Input: part model. Units: mm. Frame: model coordinates. A direction names the side the tool comes from. Round coordinates to 2 decimals unless told otherwise and drop trailing zeros. Loops run counter-clockwise (first coordinate to the right, second up) from the corner with the lowest first, then second, coordinate; pieces in that order, holes last. Notation, with made-up numbers: (45.5, 40.25) - (76.5, 40.25) arc R28 cw to (76.5, 79.25) - close; hole circle Ø8 at (-31, -33.75). An arc over 180 degrees is marked (long way). Use CSV: the item, a comma, the result in double quotes. Start each with the question number.
1. Material intervals for probe 1 along X at (y, z) = (40.5, 3.4); probe 2 along Y at (x, z) = (111.5, 3.4); probe 3 along Y at (x, z) = (22.5, 1.1), sorted ascending. Write a range as from..to.
2. Cut plane A-A (y = 37). Return loops of the section in (x, z), and give its area (3 significant figures).
3. Access query for faces 5 (the flat face through (135, -4.8, 3)), 6 (the flat face through (120, 42, 3)), 7 (the flat face through (128.725, 19.699, 2.465)). Directions: +Z, -Z, +X, -X, +Y, -Y. A direction counts if a zero-diameter tool reaches every point of the face in a straight line with its end or side. Return the directions, or none.
4. Cut plane C-C (x = 137.5). Return loops of the section in (y, z), and give its area (3 significant figures).
5. Cut plane B-B (x = 83.5). Return loops of the section in (y, z), and give its area (3 significant figures).
6. Pull-direction query (Y, two-part tool) for faces 1 (the flat face through (45, 0, 2)), 2 (the cylindrical face through (13.3, 35.5, 2.5)), 3 (the flat face through (30, 42, 3)), 4 (the flat face through (105, 40, 2)); classes: +Y half, -Y half, draft (parallel to the pull), parting line (faces both ways), or undercut.
7. Pin query (flat end, axial travel): P1, Ø2, axis at x = 32.5, z = 4.5, coming from the -Y side; P2, Ø1.5, axis at x = 105, z = 3.5, coming from the +Y side. Return the tip coordinate at first contact, or that it passes through.
8. Cut plane D-D (z = 3.75). Give the number of separate pieces and of enclosed holes in the cut face, and give its area (3 significant figures).
```python
from build123d import *

# Parameters (mm, degrees)
SKETCH_1_W          = 150
SKETCH_1_H          = 40
EXTRUDE_1_DEPTH     = 5
SKETCH_2_W          = 30
SKETCH_2_H          = 4.8
EXTRUDE_2_DEPTH     = 5
SKETCH_3_R          = 1.1
CUT_EXTRUDE_1_DEPTH = 5
FILLET_1_R          = 1
CUT_EXTRUDE_2_DEPTH = 10
FILLET_2_R          = 1.1
HOLE_WIZARD_M3_1_D  = 3.4


with BuildPart() as part:
    # 草图1 → 凸台-拉伸1 (new body)
    with BuildSketch(Plane.XY):
        with Locations((75, 20)):
            Rectangle(SKETCH_1_W, SKETCH_1_H)
    extrude(amount=EXTRUDE_1_DEPTH)

    # 草图2 → 凸台-拉伸2 (add)
    with BuildSketch(Plane.XY.offset(5)):
        with Locations((15, 42.4)):
            Rectangle(SKETCH_2_W, SKETCH_2_H)
        with Locations((75, 42.4)):
            Rectangle(SKETCH_2_W, SKETCH_2_H)
        with Locations((135, 42.4)):
            Rectangle(SKETCH_2_W, SKETCH_2_H)
        with Locations((15, -2.4)):
            Rectangle(SKETCH_2_W, SKETCH_2_H)
        with Locations((75, -2.4)):
            Rectangle(SKETCH_2_W, SKETCH_2_H)
        with Locations((135, -2.4)):
            Rectangle(SKETCH_2_W, SKETCH_2_H)
    extrude(amount=-EXTRUDE_2_DEPTH)

    # 草图3 → 切除-拉伸1 (cut)
    with BuildSketch(Plane.XY.offset(5)):
        with Locations((30, 40)):
            Circle(SKETCH_3_R)
        with Locations((60, 40)):
            Circle(SKETCH_3_R)
        with Locations((90, 40)):
            Circle(SKETCH_3_R)
        with Locations((120, 40)):
            Circle(SKETCH_3_R)
        with Locations((30, 0)):
            Circle(SKETCH_3_R)
        with Locations((60, 0)):
            Circle(SKETCH_3_R)
        with Locations((90, 0)):
            Circle(SKETCH_3_R)
        with Locations((120, 0)):
            Circle(SKETCH_3_R)
    extrude(amount=-CUT_EXTRUDE_1_DEPTH, mode=Mode.SUBTRACT)

    # 圆角1
    fillet_1_edges = [part.edges().sort_by_distance(p)[0] for p in [
        (0, 44.8, 2.5),
        (30, 44.8, 2.5),
        (60, 44.8, 2.5),
        (90, 44.8, 2.5),
        (150, 44.8, 2.5),
        (120, 44.8, 2.5),
        (0, -4.8, 2.5),
        (30, -4.8, 2.5),
        (60, -4.8, 2.5),
        (90, -4.8, 2.5),
        (120, -4.8, 2.5),
        (150, -4.8, 2.5),
    ]]
    fillet(fillet_1_edges, radius=FILLET_1_R)

    # 草图5 → 切除-拉伸2 (cut)
    with BuildSketch(Plane(origin=(0, 0, 0), x_dir=(-1, 0, 0), z_dir=(0, 0, -1))):
        Polygon((-114.766536075, 32), (-118.9, 32), (-142, 32), (-142, 8), align=None)
        Polygon((-102.666666667, 8), (-102.666666667, 32), (-129.900130591, 8), align=None)
        Polygon((-67.433202742, 8), (-94.666666667, 32), (-94.666666667, 8), align=None)
        Polygon((-8, 32), (-35.233463925, 32), (-8, 8), align=None)
        Polygon((-55.333333333, 32), (-82.566797258, 32), (-55.333333333, 8), align=None)
        Polygon((-20.099869409, 8), (-47.333333333, 32), (-47.333333333, 8), align=None)
    extrude(amount=-CUT_EXTRUDE_2_DEPTH, mode=Mode.SUBTRACT)

    # 圆角2
    fillet_2_edges = [part.edges().sort_by_distance(p)[0] for p in [
        (55.333333333, 8, 2.5),
        (82.566797258, 32, 2.5),
        (55.333333333, 32, 2.5),
        (8, 8, 2.5),
        (35.233463925, 32, 2.5),
        (8, 32, 2.5),
        (94.666666667, 32, 2.5),
        (67.433202742, 8, 2.5),
        (94.666666667, 8, 2.5),
        (102.666666667, 32, 2.5),
        (102.666666667, 8, 2.5),
        (129.900130591, 8, 2.5),
        (47.333333333, 32, 2.5),
        (20.099869409, 8, 2.5),
        (47.333333333, 8, 2.5),
        (142, 8, 2.5),
        (142, 32, 2.5),
        (114.766536075, 32, 2.5),
    ]]
    fillet(fillet_2_edges, radius=FILLET_2_R)

    # M3 间隙孔1 (through all)
    with Locations(Plane(origin=(0, 0, 0), x_dir=(-1, 0, 0), z_dir=(0, 0, -1))):
        with Locations((-137.5, 37), (-127.5, 37), (-22.5, 37), (-12.5, 37), (-137.5, 3), (-127.5, 3), (-22.5, 3), (-12.5, 3)):
            Hole(HOLE_WIZARD_M3_1_D / 2)


solid = part.part
```
Established:
1,probe 1,"x = 0..29.02, 60.98..89.02, 120.98..150"
1,probe 2,"y = 0..8, 24.22..40"
1,probe 3,"y = -4.8..1.3, 4.7..8.13, 10.12..20.78, 32..35.3, 38.7..44.8"
2,outline,"(0, 0) - (10.8, 0) - (10.8, 5) - (0, 5) - close; (14.2, 0) - (20.8, 0) - (20.8, 5) - (14.2, 5) - close; (24.2, 0) - (125.8, 0) - (125.8, 5) - (24.2, 5) - close; (129.2, 0) - (135.8, 0) - (135.8, 5) - (129.2, 5) - close; (139.2, 0) - (150, 0) - (150, 5) - (139.2, 5) - close"
2,area,"682 mm2"
3,face 5,"+Z, -Z, +X, -X, -Y"
3,face 6,"+Z, -Z, +Y"
3,face 7,"+Z, -Z"
4,outline,"(-4.8, 0) - (1.3, 0) - (1.3, 5) - (-4.8, 5) - close; (4.7, 0) - (11.97, 0) - (11.97, 5) - (4.7, 5) - close; (32, 0) - (35.3, 0) - (35.3, 5) - (32, 5) - close; (38.7, 0) - (44.8, 0) - (44.8, 5) - (38.7, 5) - close"
4,area,"114 mm2"
5,outline,"(-4.8, 0) - (8, 0) - (8, 5) - (-4.8, 5) - close; (22.16, 0) - (44.8, 0) - (44.8, 5) - (22.16, 5) - close"
5,area,"177 mm2"
6,face 1,"-Y half"
6,face 2,"undercut"
6,face 3,"draft"
6,face 4,"+Y half"
7,P1,"stops at y = 0"
7,P2,"stops at y = 40"
8,separate pieces,"1"
8,enclosed holes,"14"
8,area,"4,820 mm2"
